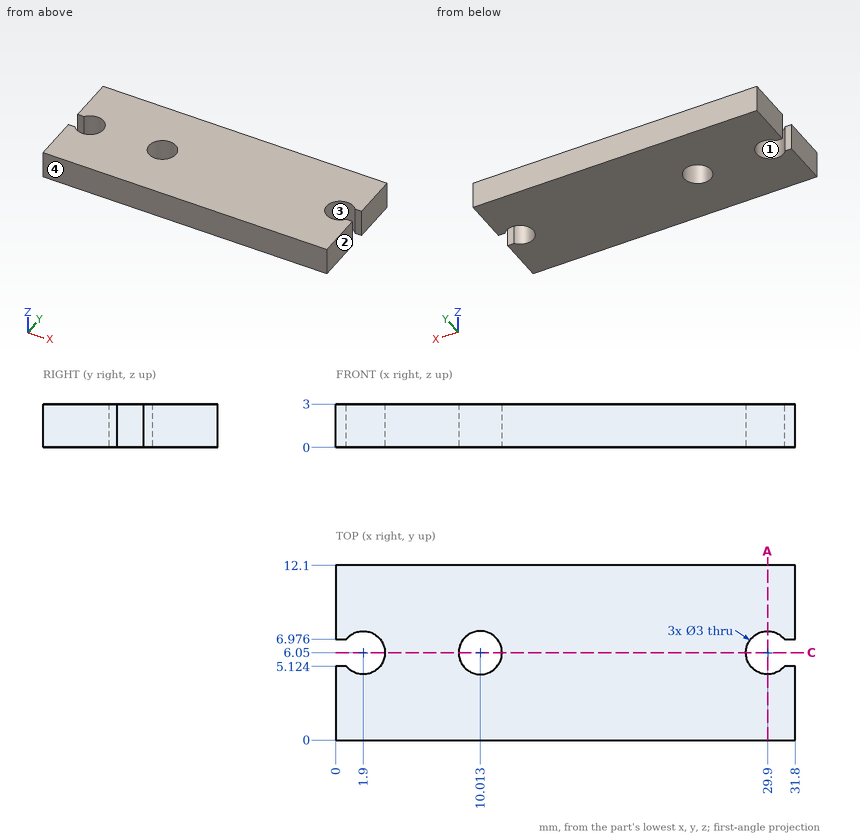
For this review, use the dimensioned drawing (mm, ordinates from the lowest corner) and the shaded views. Give positions to 0.01 mm unless a question says otherwise; leave off trailing zeros. Write each loop counter-clockwise with the first axis right and the second up, starting at its lowest first coordinate (ties: lowest second). Pieces come first, ordered by that corner, then holes. Notation, with made-up numbers: M 69,67 L 82,67 A28 cw 82,91 Z; hole C 31,-26 d8. An arc over 180 degrees is marked long. Answer as a JSON object with one key per item and string values. Group by question number.
Item 1: Consider section A-A on x = 29.9. Write out the cut boundary in (y, z).
Item 2: For probe 1 along Y at (x, z) = (1.9, 1.25); probe 2 along X at (y, z) = (6, 2.25), list the stretches that pass through material, from the lowest coordinate up. Write a range as [from, to].
Item 3: Draft analysis for pull direction Y (two halves, no side actions). For the marked faces 1, 2, 3 and 4, state which applies: +Y half, -Y half, draft (parallel to the pull), parting line (faces both ways), or undercut.
Item 4: Consider section C-C on y = 6.05. Write out the cut boundary in (x, z).
Check result:
{
 "1": {"outline": "M 0,0 L 4.55,0 L 4.55,3 L 0,3 Z; M 7.55,0 L 12.1,0 L 12.1,3 L 7.55,3 Z"},
 "2": {"probe 1": "y = [0, 4.55], [7.55, 12.1]", "probe 2": "x = [3.4, 8.51], [11.51, 28.4]"},
 "3": {"face 1": "undercut", "face 2": "draft", "face 3": "undercut", "face 4": "-Y half"},
 "4": {"outline": "M 3.4,0 L 8.51,0 L 8.51,3 L 3.4,3 Z; M 11.51,0 L 28.4,0 L 28.4,3 L 11.51,3 Z"}
}
